Could you check a few things on this model? Use its own coordinates, in mm. Give positions to 0.01 mm unless a question says otherwise; leave off trailing zeros. Write each loop counter-clockwise with the first axis right and the second up, starting at its lowest first coordinate (ties: lowest second). Pieces come first, ordered by that corner, then holes. Notation, with made-up numbers: (-19, -30.5) - (38, -30.5) arc R34 cw to (38, 3.5) - close; hole circle Ø3 at (87, 16.5). An arc over 180 degrees is marked (long way). Answer in a Markdown table with one row per item.
from build123d import *

# Parameters (mm, degrees)
EXTRUDE_1_DEPTH     = 3.6
SKETCH_2_W          = 210
SKETCH_2_H          = 50
CUT_EXTRUDE_1_DEPTH = 10


with BuildPart() as part:
    # 草图1 → 凸台-拉伸1 (new body)
    with BuildSketch(Plane.XY):
        Polygon((140, -75), (105, -75), (105, -78.6), (35, -78.6), (35, -75), (-35, -75), (-35, -78.6), (-105, -78.6), (-105, -75), (-140, -75), (-140, -56.25), (-136.4, -56.25), (-136.4, -18.75), (-140, -18.75), (-140, 18.75), (-136.4, 18.75), (-136.4, 56.25), (-140, 56.25), (-140, 75), (-105, 75), (-105, 78.6), (-35, 78.6), (-35, 75), (35, 75), (35, 78.6), (105, 78.6), (105, 75), (140, 75), (140, 56.25), (136.4, 56.25), (136.4, 18.75), (140, 18.75), (140, -18.75), (136.4, -18.75), (136.4, -56.25), (140, -56.25), align=None)
    extrude(amount=EXTRUDE_1_DEPTH)

    # 草图2 → 切除-拉伸1 (cut)
    with BuildSketch(Plane.XY.offset(3.6)):
        with Locations((0, -13.6)):
            Rectangle(SKETCH_2_W, SKETCH_2_H)
    extrude(amount=-CUT_EXTRUDE_1_DEPTH, mode=Mode.SUBTRACT)


solid = part.part
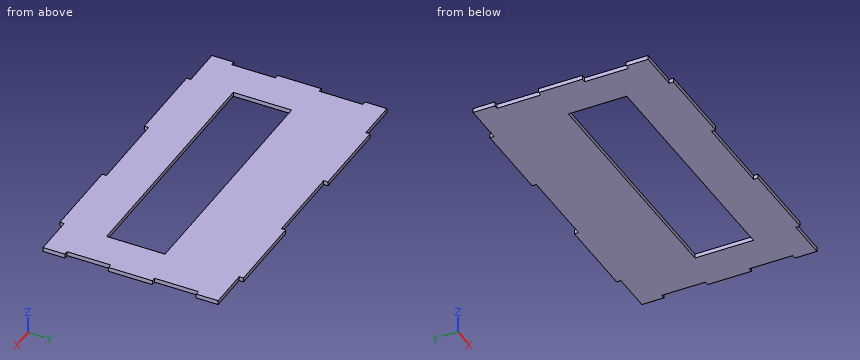
1) Imagine slicing it at A-A (x = 87). List the corners of the cut face in (y, z) for me, then the cut area to 3 significant figures.
Check values:
| item | result |
|---|---|
| outline | (-78.6, 0) - (-38.6, 0) - (-38.6, 3.6) - (-78.6, 3.6) - close; (11.4, 0) - (78.6, 0) - (78.6, 3.6) - (11.4, 3.6) - close |
| area | 386 mm2 |
2) If I drill on line 1 (X direction, y = 10.5, z = 1.3); line 2 (X direction, y = -23, z = 2.65); line 3 (Y direction, x = -43.5, z = 0.2), over which ranges is the centre line in solid material (lowest first)?
Check values:
| item | result |
|---|---|
| line 1 | x = -140 to -105, 105 to 140 |
| line 2 | x = -136.4 to -105, 105 to 136.4 |
| line 3 | y = -78.6 to -38.6, 11.4 to 78.6 |
3) Imagine slicing it at C-C (y = 26.5). List the corners of the cut face in (x, z) for me, then the cut area to 3 significant figures.
Check values:
| item | result |
|---|---|
| outline | (-136.4, 0) - (136.4, 0) - (136.4, 3.6) - (-136.4, 3.6) - close |
| area | 982 mm2 |
4) Imagine slicing it at D-D (x = 117). List the corners of the cut face in (y, z) for me, then the cut area to 3 significant figures.
Check values:
| item | result |
|---|---|
| outline | (-75, 0) - (75, 0) - (75, 3.6) - (-75, 3.6) - close |
| area | 540 mm2 |
5) Imagine slicing it at B-B (y = -33.5). List the corners of the cut face in (x, z) for me.
Check values:
| item | result |
|---|---|
| outline | (-136.4, 0) - (-105, 0) - (-105, 3.6) - (-136.4, 3.6) - close; (105, 0) - (136.4, 0) - (136.4, 3.6) - (105, 3.6) - close |
6) Will these pins go through, and if not, where does the flat tip stop? P1, Ø1.8, axis at y = 33, z = 2.5, coming from the +X side; P2, Ø1.8, axis at y = 76.5, z = 2, coming from the +X side; P3, Ø1.1, axis at x = -123.5, z = 1.5, coming from the -Y side.
Check values:
| item | result |
|---|---|
| P1 | stops at x = 136.4 |
| P2 | stops at x = 105 |
| P3 | stops at y = -75 |
